Can you work these out from the model? Positions are in its coordinate system, mm. A direction names the side the tool comes from. Give positions to 0.01 mm unless a question says otherwise; leave off trailing zeros. Order: outer loops, then holes, each group sorted by start corner. A loop starts at its lowest first (then second) coordinate and runs counter-clockwise, first axis right, second up.
```python
from build123d import *

# Parameters (mm, degrees)
SKETCH2_R           = 23
SKETCH2_R_2         = 1.5
BOSS_EXTRUDE1_DEPTH = 1.5


with BuildPart() as part:
    # Sketch2 → Boss-Extrude1 (new body)
    with BuildSketch(Plane.XY):
        with BuildLine():
            Line((26, -3.1), (28, -3.1))
            ThreePointArc((28, -3.1), (31.1, 0), (28, 3.1))
            Line((28, 3.1), (26, 3.1))
            ThreePointArc((26, 3.1), (25.713286425, 3.086712705), (25.429030688, 3.046964726))
            ThreePointArc((25.429030688, 3.046964726), (18.109660347, 18.109660347), (3.046964726, 25.429030688))
            ThreePointArc((3.046964726, 25.429030688), (3.086712705, 25.713286425), (3.1, 26))
            Line((3.1, 26), (3.1, 28))
            ThreePointArc((3.1, 28), (0, 31.1), (-3.1, 28))
            Line((-3.1, 28), (-3.1, 26))
            ThreePointArc((-3.1, 26), (-3.086712705, 25.713286425), (-3.046964726, 25.429030688))
            ThreePointArc((-3.046964726, 25.429030688), (-18.109660347, 18.109660347), (-25.429030688, 3.046964726))
            ThreePointArc((-25.429030688, 3.046964726), (-25.713286425, 3.086712705), (-26, 3.1))
            Line((-26, 3.1), (-28, 3.1))
            ThreePointArc((-28, 3.1), (-31.1, 0), (-28, -3.1))
            Line((-28, -3.1), (-26, -3.1))
            ThreePointArc((-26, -3.1), (-25.713286425, -3.086712705), (-25.429030688, -3.046964726))
            ThreePointArc((-25.429030688, -3.046964726), (-18.109660347, -18.109660347), (-3.046964726, -25.429030688))
            ThreePointArc((-3.046964726, -25.429030688), (-3.086712705, -25.713286425), (-3.1, -26))
            Line((-3.1, -26), (-3.1, -28))
            ThreePointArc((-3.1, -28), (0, -31.1), (3.1, -28))
            Line((3.1, -28), (3.1, -26))
            ThreePointArc((3.1, -26), (3.086712705, -25.713286425), (3.046964726, -25.429030688))
            ThreePointArc((3.046964726, -25.429030688), (18.109660347, -18.109660347), (25.429030688, -3.046964726))
            ThreePointArc((25.429030688, -3.046964726), (25.713286425, -3.086712705), (26, -3.1))
        make_face()
        Circle(SKETCH2_R, mode=Mode.SUBTRACT)
        with Locations((-28, 0)):
            Circle(SKETCH2_R_2, mode=Mode.SUBTRACT)
        with Locations((0, 28)):
            Circle(SKETCH2_R_2, mode=Mode.SUBTRACT)
        with Locations((28, 0)):
            Circle(SKETCH2_R_2, mode=Mode.SUBTRACT)
        with Locations((0, -28)):
            Circle(SKETCH2_R_2, mode=Mode.SUBTRACT)
    extrude(amount=BOSS_EXTRUDE1_DEPTH)


solid = part.part
```
1) Which directions (+Z, -Z, +X, -X, +Y, -Y) give clear straight access to the entire face, cutting with the end or side of a thin tool? Please do faces 1 (the face through (27, 3.1, 1)), 2 (the face through (-29.5, 0.07, 0.74)), 3 (the face through (-3.1, 27, 1)).
2) Suppose I cut it at B-B (x = -19). Please give me the cut outline in (y, z), and give its area (3 significant figures).
3) If I drill on line 1 (Y direction, x = 0, z = 1.15); line 2 (Y direction, x = -28, z = 0.45); line 3 (X direction, y = -1, z = 0.3), over which ranges is the centre line in solid material (lowest first)?
4) We'd pull the mould along Y, two halves only. Please class faces 4 (the face through (3.1, -27, 1)), 5 (the face through (0.1, 31.1, 0.7)), 6 (the face through (31.1, -0.1, 0.7)), 7 (the face through (-2.994, 22.804, 0.74)): +Y half, -Y half, draft (parallel to the pull), parting line (faces both ways), or undercut.
5) Suppose I cut it at A-A (y = 0). Please give me the cut outline in (x, z).
6) Suppose I cut it at D-D (y = -12). Please give me the cut outline in (x, z), and give its area (3 significant figures).
7) I'm going to push flat-ended pins straight in: pin 1 Ø0.8 at (x, z) = (27.5, 0.5) entering from +Y; pin 2 Ø1.8 at (x, y) = (0, 28) entering from -Z; pin 3 Ø0.8 at (y, z) = (-26.5, 0.5) entering from +X. Where does each tip first touch, or does it pass through?
8) Suppose I cut it at C-C (z = 0.75). Give the number of separate pieces and of enclosed holes in the cut face, and give its area (3 significant figures).
Results:
1. face 1: +Z, -Z, +X, +Y
1. face 2: +Z, -Z
1. face 3: +Z, -Z, -X, +Y
2. outline: (-17.17, 0) - (-12.96, 0) - (-12.96, 1.5) - (-17.17, 1.5) - close; (12.96, 0) - (17.17, 0) - (17.17, 1.5) - (12.96, 1.5) - close
2. area: 12.6 mm2
3. line 1: y = -31.1 to -29.5, -26.5 to -23, 23 to 26.5, 29.5 to 31.1
3. line 2: y = -3.1 to -1.5, 1.5 to 3.1
3. line 3: x = -30.93 to -29.12, -26.88 to -22.98, 22.98 to 26.88, 29.12 to 30.93
4. face 4: draft
4. face 5: +Y half
4. face 6: parting line
4. face 7: undercut
5. outline: (-31.1, 0) - (-29.5, 0) - (-29.5, 1.5) - (-31.1, 1.5) - close; (-26.5, 0) - (-23, 0) - (-23, 1.5) - (-26.5, 1.5) - close; (23, 0) - (26.5, 0) - (26.5, 1.5) - (23, 1.5) - close; (29.5, 0) - (31.1, 0) - (31.1, 1.5) - (29.5, 1.5) - close
6. outline: (-22.63, 0) - (-19.62, 0) - (-19.62, 1.5) - (-22.63, 1.5) - close; (19.62, 0) - (22.63, 0) - (22.63, 1.5) - (19.62, 1.5) - close
6. area: 9.01 mm2
7. pin 1: stops at y = 3.1
7. pin 2: passes through
7. pin 3: stops at x = 3.1
8. separate pieces: 1
8. enclosed holes: 5
8. area: 492 mm2
